The listing builds one solid part. Answer for the finished solid, in the listing's coordinates (mm). A direction names the side the tool comes from. Coordinates: 2 decimals unless noted, no trailing zeros. Order: outer loops, then holes, each group sorted by start corner. A loop starts at its lowest first (then second) coordinate and runs counter-clockwise, first axis right, second up. Notation, with made-up numbers: (-20.5, 30.25) - (-10.5, 30.25) arc R26 ccw to (-10.5, 63.25) - close; hole circle Ø2 at (64.25, 8). An arc over 180 degrees is marked (long way). Use a Markdown table: item, result. Add a question column.
Item 1: The part is cut by section B-B, the plane z = 36. Give the vertices of the cut face in (x, y).
Item 2: Flat-ended cylindrical pins translate along their axes: P1, Ø8, axis at x = -9.5, y = 33.5, coming from the +Z side; P2, Ø2.5, axis at y = 20.5, z = 29.5, coming from the +X side; P3, Ø5, axis at x = -15, y = 25.5, coming from the -Z side; P4, Ø3, axis at x = -1, z = 28.5, coming from the +Y side. Find the tip coordinate at first contact, or state that the pin passes through.
Item 3: Find the intervals of material crossed by line 1 along X through (y, z) = (17.8, 81.5); line 2 along Z through (x, y) = (-34.5, 16); line 3 along X through (y, z) = (25.75, 39.5), in increasing order.
Item 4: For faces 4 (the flat face through (33.9, 23.512, 32.2)), 5 (the flat face through (-6, 25, 66)), 6 (the flat face through (-4, 20, -12)), determine the directions among +Z, -Z, +X, -X, +Y, -Y from which every point of the face is accessible in a straight line to the end or side of a thin tool.
Item 5: The mould has two halves that part along X. Classify faces 1 (the flat face through (-1, 14.012, 27)), 2 (the flat face through (-40.1, 23.1, 4.7)), 3 (the cylindrical face through (14.049, 16.547, 57.214)): released by +X, released by -X, zero draft, split by the parting line, or undercut.
Item 6: The part is cut by section A-A, the plane x = 19. Give the vertices of the cut face in (y, z), then the cut area to 3 significant figures.
Item 7: The part is cut by section C-C, the plane z = 22. Give the vertices of the cut face in (x, y), then the cut area to 3 significant figures.
from build123d import *

# Parameters (mm, degrees)
SKETCH003_R          = 9
SKETCH003_R_2        = 3.125
PAD_DEPTH            = 18
SKETCH005_R          = 2.5
POCKET_DEPTH         = 19.001
POCKET_DEPTH_BACK    = 0.001
POCKET007_DEPTH      = 13
SKETCH025_R          = 1.6
POCKET008_DEPTH      = 18.001
POCKET008_DEPTH_BACK = 0.001
SKETCH026_R          = 3.65
POCKET009_DEPTH      = 3.4
SKETCH075_R          = 2.5
POCKET038_DEPTH      = 18.001
SKETCH033_W          = 8.1
SKETCH033_H          = 8.1
POCKET011_DEPTH      = 7.251
SKETCH030_W          = 8.1
SKETCH030_H          = 8.1
POCKET010_DEPTH      = 9.5
SKETCH034_W          = 20.4
SKETCH034_H          = 40.4
POCKET012_DEPTH      = 16
SKETCH035_R          = 2.63
POCKET013_DEPTH      = 52.001
POCKET013_DEPTH_BACK = 32.001
SKETCH036_R          = 5.25
POCKET014_DEPTH      = 46.001
SKETCH037_R          = 5.25
POCKET015_DEPTH      = 10.001
PAD032_DEPTH         = 6
POCKET053_DEPTH      = 20
SKETCH106_R          = 2.1
POCKET054_DEPTH      = 0.001
POCKET054_DEPTH_BACK = 24.001


with BuildPart() as obj1:
    # Sketch003 → Pad (new body)
    with BuildSketch(Plane.XZ.offset(-1)):
        with BuildLine():
            ThreePointArc((-32, 40.35), (-39.331308, 37.150876), (-41.971864, 29.600384))
            Line((-41.971864, 29.600384), (-38.171864, -20.949616))
            ThreePointArc((-38.171864, -20.949616), (-36.159823, -26.253199), (-31.586604, -29.609087))
            Line((-31.586604, -29.609087), (-3.386604, -39.759087))
            ThreePointArc((-3.386604, -39.759087), (3.616839, -39.673008), (8.846019, -35.01347))
            Line((40.846019, 25.68653), (8.846019, -35.01347))
            ThreePointArc((40.846019, 25.68653), (41.707219, 27.947937), (42, 30.35))
            Line((42, 30.35), (42, 40.35))
            Line((42, 87), (42, 40.35))
            ThreePointArc((42, 87), (40.535534, 90.535534), (37, 92))
            Line((-5, 92), (37, 92))
            ThreePointArc((-5, 92), (-8.535534, 90.535534), (-10, 87))
            Line((-10, 79.35), (-10, 87))
            Line((-10, 79.35), (-27, 79.35))
            ThreePointArc((-27, 79.35), (-29.12132, 78.47132), (-30, 76.35))
            Line((-30, 76.35), (-30, 60.35))
            ThreePointArc((-30, 60.35), (-29.12132, 58.22868), (-27, 57.35))
            Line((-10, 57.35), (-27, 57.35))
            Line((-10, 40.35), (-10, 57.35))
            Line((-32, 40.35), (-10, 40.35))
        make_face()
        with Locations((16, 66)):
            Circle(SKETCH003_R, mode=Mode.SUBTRACT)
        with Locations((-18, 10)):
            Circle(SKETCH003_R_2, mode=Mode.SUBTRACT)
        with Locations((-18, -10)):
            Circle(SKETCH003_R_2, mode=Mode.SUBTRACT)
    extrude(amount=-PAD_DEPTH)

    # Sketch005 → Pocket (cut, two sides)
    with BuildSketch(Plane.XZ) as pocket_sk:
        with Locations((-32, 30.35)):
            Circle(SKETCH005_R)
        with Locations((32, 30.35)):
            Circle(SKETCH005_R)
        with Locations((0, -30.35)):
            Circle(SKETCH005_R)
    extrude(amount=-POCKET_DEPTH, mode=Mode.SUBTRACT)
    extrude(pocket_sk.sketch, amount=POCKET_DEPTH_BACK, mode=Mode.SUBTRACT)

    with BuildSketch(Plane(origin=(16, 14, 66), x_dir=(-1, 0, 0), z_dir=(0, 1, 0))):
        with BuildLine():
            Line((-20, 22), (20, 22))
            ThreePointArc((22, 20), (21.414214, 21.414214), (20, 22))
            Line((22, 20), (22, -20))
            ThreePointArc((20, -22), (21.414214, -21.414214), (22, -20))
            Line((20, -22), (-20, -22))
            ThreePointArc((-22, -20), (-21.414214, -21.414214), (-20, -22))
            Line((-22, -20), (-22, 20))
            ThreePointArc((-20, 22), (-21.414214, 21.414214), (-22, 20))
        make_face()
    extrude(amount=-POCKET007_DEPTH, mode=Mode.SUBTRACT)

    with BuildSketch(Plane(origin=(16, 19, 66), x_dir=(-1, 0, 0), z_dir=(0, 1, 0))) as pocket008_sk:
        with Locations((-15.5, 15.5)):
            Circle(SKETCH025_R)
        with Locations((15.5, 15.5)):
            Circle(SKETCH025_R)
        with Locations((-15.5, -15.5)):
            Circle(SKETCH025_R)
        with Locations((15.5, -15.5)):
            Circle(SKETCH025_R)
    extrude(amount=-POCKET008_DEPTH, mode=Mode.SUBTRACT)
    extrude(pocket008_sk.sketch, amount=POCKET008_DEPTH_BACK, mode=Mode.SUBTRACT)

    with BuildSketch(Plane(origin=(16, 19, 66), x_dir=(-1, 0, 0), z_dir=(0, 1, 0))):
        with Locations((-15.5, 15.5)):
            Circle(SKETCH026_R)
        with Locations((15.5, 15.5)):
            Circle(SKETCH026_R)
        with Locations((-15.5, -15.5)):
            Circle(SKETCH026_R)
        with Locations((15.5, -15.5)):
            Circle(SKETCH026_R)
    extrude(amount=-POCKET009_DEPTH, mode=Mode.SUBTRACT)

    with BuildSketch(Plane(origin=(8, 19, 36), x_dir=(-1, 0, 0), z_dir=(0, 1, 0))):
        with Locations((-10, 0)):
            Circle(SKETCH075_R)
        with Locations((10, 0)):
            Circle(SKETCH075_R)
    extrude(amount=-POCKET038_DEPTH, mode=Mode.SUBTRACT)

    with BuildSketch(Plane(origin=(8, 8.25, 36), x_dir=(-1, 0, 0), z_dir=(0, 1, 0))):
        with Locations((-10, 0)):
            Rectangle(SKETCH033_W, SKETCH033_H)
        with Locations((10, 0)):
            Rectangle(SKETCH033_W, SKETCH033_H)
    extrude(amount=-POCKET011_DEPTH, mode=Mode.SUBTRACT)

    # Sketch030 (on DatumPlane) → Pocket010 (cut)
    with BuildSketch(Plane(origin=(0, 19, 0), x_dir=(-1, 0, 0), z_dir=(0, 1, 0))):
        with Locations((-32, 30.35)):
            Rectangle(SKETCH030_W, SKETCH030_H)
        with Locations((32, 30.35)):
            Rectangle(SKETCH030_W, SKETCH030_H)
        with Locations((0, -30.35)):
            Rectangle(SKETCH030_W, SKETCH030_H)
    extrude(amount=-POCKET010_DEPTH, mode=Mode.SUBTRACT)

    # Sketch034 (on DatumPlane) → Pocket012 (cut)
    with BuildSketch(Plane(origin=(0, 19, 0), x_dir=(-1, 0, 0), z_dir=(0, 1, 0))):
        with Locations((18, 0)):
            Rectangle(SKETCH034_W, SKETCH034_H)
    extrude(amount=-POCKET012_DEPTH, mode=Mode.SUBTRACT)

    # Sketch035 → Pocket013 (cut, two sides)
    with BuildSketch(Plane(origin=(10, 11, 0), x_dir=(0, 1, 0), z_dir=(1, 0, 0))) as pocket013_sk:
        with Locations((0, 10)):
            Circle(SKETCH035_R)
        with Locations((0, -10)):
            Circle(SKETCH035_R)
    extrude(amount=-POCKET013_DEPTH, mode=Mode.SUBTRACT)
    extrude(pocket013_sk.sketch, amount=POCKET013_DEPTH_BACK, mode=Mode.SUBTRACT)

    # Sketch036 → Pocket014 (cut, through all)
    with BuildSketch(Plane(origin=(-4, 11, 0), x_dir=(0, 1, 0), z_dir=(1, 0, 0))):
        with Locations((0, 10)):
            Circle(SKETCH036_R)
        with Locations((0, -10)):
            Circle(SKETCH036_R)
    extrude(amount=POCKET014_DEPTH, mode=Mode.SUBTRACT)

    # Sketch037 → Pocket015 (cut, through all)
    with BuildSketch(Plane(origin=(-32, 11, 0), x_dir=(0, 1, 0), z_dir=(1, 0, 0))):
        with Locations((0, 10)):
            Circle(SKETCH037_R)
        with Locations((0, -10)):
            Circle(SKETCH037_R)
    extrude(amount=-POCKET015_DEPTH, mode=Mode.SUBTRACT)

    # Sketch104 → Pad032 (join)
    with BuildSketch(Plane.XZ.offset(-1)):
        with BuildLine():
            Line((-13, 79.35), (-27, 79.35))
            ThreePointArc((-27, 79.35), (-29.12132, 78.47132), (-30, 76.35))
            Line((-30, 76.35), (-30, 60.35))
            ThreePointArc((-30, 60.35), (-29.12132, 58.22868), (-27, 57.35))
            Line((-13, 57.35), (-27, 57.35))
            ThreePointArc((-13, 57.35), (-10.87868, 58.22868), (-10, 60.35))
            Line((-10, 76.35), (-10, 60.35))
            ThreePointArc((-10, 76.35), (-10.87868, 78.47132), (-13, 79.35))
        make_face()
    extrude(amount=PAD032_DEPTH)

    # Sketch105 → Pocket053 (cut)
    with BuildSketch(Plane.XZ.offset(-19)):
        Polygon((-20, 76.128175), (-12.221825, 68.35), (-20, 60.571825), (-27.778175, 68.35), align=None)
    extrude(amount=POCKET053_DEPTH, mode=Mode.SUBTRACT)

    # Sketch106 → Pocket054 (cut, two sides)
    with BuildSketch(Plane.XZ.offset(-19)) as pocket054_sk:
        with Locations((-20, 68.35)):
            Circle(SKETCH106_R)
    extrude(amount=-POCKET054_DEPTH, mode=Mode.SUBTRACT)
    extrude(pocket054_sk.sketch, amount=POCKET054_DEPTH_BACK, mode=Mode.SUBTRACT)


with BuildPart() as obj2:
    # Part__Mirroring002: instance of obj1
    add(obj1.part.mirror(Plane(origin=(2.8e-05, 16.506189, 25.826885), x_dir=(1, 0, 0), z_dir=(0, 1, 0))))


solid = obj2.part
Solution:
| question | item | result |
|---|---|---|
| 1 | outline | (-40.25, 14.01) - (-4.5, 14.01) - (-4.5, 24.76) - (-6.05, 24.76) - (-6.05, 32.01) - (-40.25, 32.01) - close; (0.5, 14.01) - (15.5, 14.01) - (15.5, 24.76) - (13.95, 24.76) - (13.95, 32.01) - (2.05, 32.01) - (2.05, 24.76) - (0.5, 24.76) - close; (20.5, 14.01) - (42, 14.01) - (42, 32.01) - (22.05, 32.01) - (22.05, 24.76) - (20.5, 24.76) - close |
| 2 | P1 | stops at z = 91.94 |
| 2 | P2 | stops at x = 42 |
| 2 | P3 | stops at z = -36.48 |
| 2 | P4 | stops at y = 32.01 |
| 3 | line 1 | x = -10 to -1.1, 2.1 to 29.9, 33.1 to 42 |
| 3 | line 2 | z = -27.97 to 26.3, 34.4 to 40.03 |
| 3 | line 3 | x = -36.03 to -6.05, 2.05 to 13.95, 22.05 to 42 |
| 4 | face 4 | -Y |
| 4 | face 5 | +Y |
| 4 | face 6 | +X |
| 5 | face 1 | zero draft |
| 5 | face 2 | released by -X |
| 5 | face 3 | undercut |
| 6 | outline | (14.01, -15.75) - (32.01, -15.75) - (32.01, 31.95) - (24.76, 31.95) - (24.76, 33.71) - (14.01, 33.71) - close; (14.01, 38.29) - (24.76, 38.29) - (24.76, 40.05) - (32.01, 40.05) - (32.01, 44) - (19.01, 44) - (19.01, 57.51) - (14.01, 57.51) - close; (14.01, 74.49) - (19.01, 74.49) - (19.01, 88) - (32.01, 88) - (32.01, 92) - (14.01, 92) - close; hole circle Ø10.5 at (22.01, -10); hole circle Ø10.5 at (22.01, 10) |
| 6 | area | 1,000 mm2 |
| 7 | outline | (-41.4, 14.01) - (38.9, 14.01) - (38.9, 32.01) - (-41.4, 32.01) - close |
| 7 | area | 1,450 mm2 |
